Input: part model. Units: mm. Frame: model coordinates. Face numbers are marked on the shaded views. Give positions to 0.01 mm unless a question says otherwise; leave off trailing zeros. Order: outer loops, then holes, each group sorted by start corner. A loop starts at its lowest first (then second) coordinate and runs counter-clockwise, first axis right, second up. Notation, with made-up numbers: (88.25, 0) - (120.25, 0) arc R27 ccw to (120.25, 22) - close; hole circle Ø8 at (-11, 73). An arc over 180 degrees is marked (long way). Answer in a Markdown table with one row per item. Add a question column.
1. Section query A-A on y = 345. Return loops of the section in (x, z), and give its area (3 significant figures).
2. Section query B-B on x = 184.5. Return loops of the section in (y, z), and give its area (3 significant figures).
3. Section query C-C on y = -204. Return loops of the section in (x, z).
4. Mould query, pull axis Y, two halves, no side actions, for the marked faces 1 and 2. Classes: released by +Y, released by -Y, zero draft, split by the parting line, or undercut.
5. Section query D-D on x = 345. Count the separate pieces of the cut face and the enclosed holes in it, and give its area (3 significant figures).
6. Contact query for flat-ended pins moving along their axis: pin 1 (4 mm diameter, centred on x = 65.5, z = 25, fed in from -Y); pin 2 (3 mm diameter, centred on x = 113.5, z = 41.5, fed in from +Y); pin 3 (3 mm diameter, centred on x = -186, z = 16, fed in from +Y). Output: stop coordinate, or through.
7. Ray query, line 1 (Y direction, x = 345, z = 1.1); line 2 (Y direction, x = -8, z = 66); line 3 (Y direction, x = 0, z = 75). Return the intervals inside material, ascending. Write a range as [from, to].
```python
from build123d import *
from build123d import SkipClean  # not in build123d's __all__

# Parameters (mm, degrees)
F0_W     = 10
F0_H     = 3
F2_W     = 750
F2_H     = 750
F2_R     = 10
F3_DEPTH = 3
F6_R     = 9
F7_DEPTH = 120
F8_R     = 300
F9_DEPTH = 200


with BuildPart() as f1:
    # F0 (on Front) → F1 (revolve)
    with BuildSketch(Plane.XZ):
        Polygon((-325, 5), (-300, 5), (-300, 55), (-301, 55), (-301, 95), (-324, 95), (-324, 55), (-325, 55), align=None)
        Polygon((-10, 5), (-300, 5), (-325, 5), (-325, 2), (-10, 2), align=None)
        with Locations((-5, 3.5)):
            Rectangle(F0_W, F0_H)
    revolve(axis=Axis((0, 0, 187.9212413023), (0, 0, -1)))

    # F2 (on Top) → F3 (join)
    with BuildSketch(Plane.XY):
        Rectangle(F2_W, F2_H)
        with Locations((-345, -345)):
            Circle(F2_R, mode=Mode.SUBTRACT)
        with Locations((345, -345)):
            Circle(F2_R, mode=Mode.SUBTRACT)
        with Locations((-345, 345)):
            Circle(F2_R, mode=Mode.SUBTRACT)
        with Locations((345, 345)):
            Circle(F2_R, mode=Mode.SUBTRACT)
    extrude(amount=F3_DEPTH)

    # F4 (on Front) → F5 (revolve)
    with BuildSketch(Plane.XZ):
        Polygon((399.6194698092, 41.5098406888), (300, 50.2254149636), (299.9128442573, 49.2292202655), (399.5323140664, 40.5136459907), align=None)
    revolve(axis=Axis((412.7442754949, 0, 30.3233706049), (0.9961946981, 0, -0.0871557427)))

    # F6 (on face) → F7 (cut)
    with BuildSketch(Plane(origin=(392.9798568705, 0, -34.3812824702), x_dir=(0, 1, 0), z_dir=(0.9961946981, 0, -0.0871557427))):
        with Locations((0, 66.1810149205)):
            Circle(F6_R)
    extrude(amount=-F7_DEPTH, mode=Mode.SUBTRACT)

    # F8 (on face) → F9 (cut)
    with BuildSketch(Plane.XY.offset(5)):
        Circle(F8_R)
    with SkipClean():  # cleaning this boolean's faces spoils the solid; the shape is the same uncleaned
        extrude(amount=F9_DEPTH, mode=Mode.SUBTRACT)


solid = f1.part
```
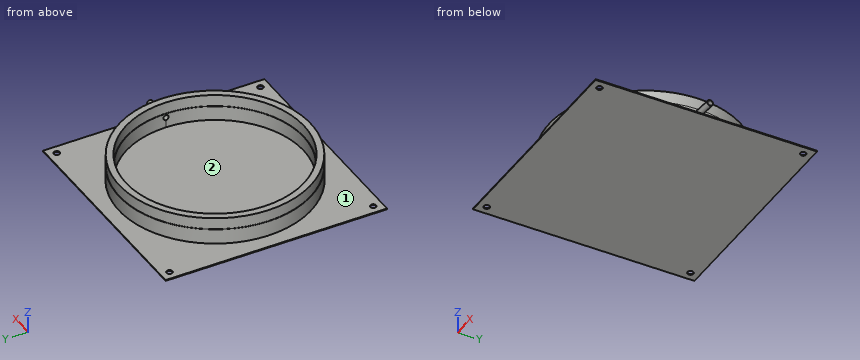
Answer:
| question | item | result |
|---|---|---|
| 1 | outline | (-375, 0) - (-355, 0) - (-355, 3) - (-375, 3) - close; (-335, 0) - (335, 0) - (335, 3) - (-335, 3) - close; (355, 0) - (375, 0) - (375, 3) - (355, 3) - close |
| 1 | area | 2,130 mm² |
| 2 | outline | (-375, 0) - (375, 0) - (375, 3) - (267.55, 3) - (267.55, 55) - (266.34, 55) - (266.34, 95) - (237.83, 95) - (237.83, 55) - (236.56, 55) - (236.56, 5) - (-236.56, 5) - (-236.56, 55) - (-237.83, 55) - (-237.83, 95) - (-266.34, 95) - (-266.34, 55) - (-267.55, 55) - (-267.55, 3) - (-375, 3) - close |
| 2 | area | 8,700 mm² |
| 3 | outline | (-375, 0) - (375, 0) - (375, 3) - (253, 3) - (253, 55) - (251.71, 55) - (251.71, 95) - (221.33, 95) - (221.33, 55) - (219.96, 55) - (219.96, 5) - (-219.96, 5) - (-219.96, 55) - (-221.33, 55) - (-221.33, 95) - (-251.71, 95) - (-251.71, 55) - (-253, 55) - (-253, 3) - (-375, 3) - close |
| 4 | face 1 | zero draft |
| 4 | face 2 | undercut |
| 5 | separate pieces | 4 |
| 5 | enclosed holes | 1 |
| 5 | area | 2,190 mm² |
| 6 | pin 1 | stops at y = -318.74 |
| 6 | pin 2 | stops at y = 305.09 |
| 6 | pin 3 | stops at y = 267.55 |
| 7 | line 1 | y = [-375, -355], [-335, 335], [355, 375] |
| 7 | line 2 | y = [-323.9, -300.89], [300.89, 323.9] |
| 7 | line 3 | y = [-324, -301], [301, 324] |
